from build123d import *

# Parameters (mm, degrees)
SKETCH1_W           = 150
SKETCH1_H           = 140
BOSS_EXTRUDE1_DEPTH = 10
SKETCH2_W           = 10.4
SKETCH2_H           = 41.4
CUT_EXTRUDE1_DEPTH  = 5
BOSS_EXTRUDE2_DEPTH = 150
SKETCH4_W           = 150
SKETCH4_H           = 10
SKETCH4_R           = 2
BOSS_EXTRUDE3_DEPTH = 5
SKETCH5_R           = 2
CUT_EXTRUDE2_DEPTH  = 6
SKETCH6_R           = 1.5
CUT_EXTRUDE3_DEPTH  = 5
SKETCH7_R           = 2.5
CUT_EXTRUDE4_DEPTH  = 2
SKETCH8_W           = 130
SKETCH8_H           = 120
CUT_EXTRUDE5_DEPTH  = 5
FILLET1_R           = 2.5


with BuildPart() as part:
    # Sketch1 → Boss-Extrude1 (new body)
    with BuildSketch(Plane(origin=(0, 0, 0), x_dir=(1, 0, 0), z_dir=(0, 1, 0))):
        Rectangle(SKETCH1_W, SKETCH1_H)
    extrude(amount=BOSS_EXTRUDE1_DEPTH)

    # Sketch2 → Cut-Extrude1 (cut)
    with BuildSketch(Plane.XZ):
        with Locations((-69.9, 0)):
            Rectangle(SKETCH2_W, SKETCH2_H)
        with Locations((69.9, 0)):
            Rectangle(SKETCH2_W, SKETCH2_H)
    extrude(amount=-CUT_EXTRUDE1_DEPTH, mode=Mode.SUBTRACT)

    # Sketch3 → Boss-Extrude2 (add)
    with BuildSketch(Plane.ZY.offset(75)):
        Polygon((-70, 13), (-70, 10), (-60, 10), (-60, 16), (-65, 16), align=None)
        Polygon((70, 10), (70, 13), (65, 16), (60, 16), (60, 10), align=None)
    extrude(amount=-BOSS_EXTRUDE2_DEPTH)

    # Sketch4 → Boss-Extrude3 (add)
    with BuildSketch(Plane(origin=(0, 10, 0), x_dir=(1, 0, 0), z_dir=(0, 1, 0))):
        with Locations((0, 55)):
            Rectangle(SKETCH4_W, SKETCH4_H)
        with Locations((-70, 55)):
            Circle(SKETCH4_R, mode=Mode.SUBTRACT)
        with Locations((70, 55)):
            Circle(SKETCH4_R, mode=Mode.SUBTRACT)
        with Locations((0, -55)):
            Rectangle(SKETCH4_W, SKETCH4_H)
        with Locations((70, -55)):
            Circle(SKETCH4_R, mode=Mode.SUBTRACT)
        with Locations((-70, -55)):
            Circle(SKETCH4_R, mode=Mode.SUBTRACT)
    extrude(amount=BOSS_EXTRUDE3_DEPTH)

    # Sketch5 → Cut-Extrude2 (cut)
    with BuildSketch(Plane(origin=(0, 15, 0), x_dir=(1, 0, 0), z_dir=(0, 1, 0))):
        with Locations((-70, 55)):
            Circle(SKETCH5_R)
        with Locations((70, 55)):
            Circle(SKETCH5_R)
        with Locations((-70, -55)):
            Circle(SKETCH5_R)
        with Locations((70, -55)):
            Circle(SKETCH5_R)
    extrude(amount=-CUT_EXTRUDE2_DEPTH, mode=Mode.SUBTRACT)

    # Sketch6 → Cut-Extrude3 (cut)
    with BuildSketch(Plane(origin=(0, 5, 0), x_dir=(-1, 0, 0), z_dir=(0, -1, 0))):
        with Locations((69.899999566, -11.999895835)):
            Circle(SKETCH6_R)
        with Locations((69.899999566, 11.999895835)):
            Circle(SKETCH6_R)
        with Locations((-69.899999566, -11.999895835)):
            Circle(SKETCH6_R)
        with Locations((-69.899999566, 11.999895835)):
            Circle(SKETCH6_R)
    extrude(amount=-CUT_EXTRUDE3_DEPTH, mode=Mode.SUBTRACT)

    # Sketch7 → Cut-Extrude4 (cut)
    with BuildSketch(Plane(origin=(0, 10, 0), x_dir=(1, 0, 0), z_dir=(0, 1, 0))):
        with Locations((-69.899999566, 11.999895835)):
            Circle(SKETCH7_R)
        with Locations((-69.899999566, -11.999895835)):
            Circle(SKETCH7_R)
        with Locations((69.899999566, -11.999895835)):
            Circle(SKETCH7_R)
        with Locations((69.899999566, 11.999895835)):
            Circle(SKETCH7_R)
    extrude(amount=-CUT_EXTRUDE4_DEPTH, mode=Mode.SUBTRACT)

    # Sketch8 → Cut-Extrude5 (cut)
    with BuildSketch(Plane(origin=(0, 15, 0), x_dir=(1, 0, 0), z_dir=(0, 1, 0))):
        Rectangle(SKETCH8_W, SKETCH8_H)
    extrude(amount=-CUT_EXTRUDE5_DEPTH, mode=Mode.SUBTRACT)

    # Fillet1
    fillet1_edges = [part.edges().sort_by_distance(p)[0] for p in [
        (-70, 10, 50),
        (70, 10, 50),
        (70, 10, -50),
        (65, 12.5, -50),
        (65, 10, -55),
        (65, 12.5, 50),
        (-65, 10, -55),
        (-65, 12.5, -50),
        (-65, 12.5, 50),
        (65, 10, 55),
        (-65, 10, 55),
        (-70, 10, -50),
    ]]
    fillet(fillet1_edges, radius=FILLET1_R)


solid = part.part
Geometry check sheet. Reference: the model listing, model coordinates, mm. A direction names the side the tool comes from. Round coordinates to 2 decimals unless told otherwise and drop trailing zeros. Order: outer loops, then holes, each group sorted by start corner. A loop starts at its lowest first (then second) coordinate and runs counter-clockwise, first axis right, second up. Notation, with made-up numbers: M -22,28 L -10,28 A22 cw -10,55 Z; hole C -12.75,51 d6. An arc over 180 degrees is marked long. Write each question's results on one line, items separated by ' | '. Start each with the question number.
1. Cross-section at A-A on x = -28. Record the boundary of the cut face in (y, z), plus the area to 4 significant figures.
2. Draft check along Z on faces 1 (the face through (70, 9, -55)), 2 (the face through (-1, 14.5, -67.5)), 3 (the face through (-1, 6, 70)). Enter one of: pulls with the +Z half, pulls with the -Z half, needs draft (parallel to the pull), parting line crosses it, or undercut.
3. Cross-section at B-B on z = -55. Record the boundary of the cut face in (x, y).
4. Cross-section at D-D on z = -0.5. Record the boundary of the cut face in (x, y), plus the area to 3 significant figures.
5. Set-up check for faces 4 (the face through (-67.515, 9.014, 11.249)), 5 (the face through (70, 5, 0)), 6 (the face through (69.9, 15, 57.2)), 7 (the face through (-70, 2, 20.7)): record each of +Z, -Z, +X, -X, +Y, -Y from which the full face is reachable in a straight line by a thin tool's end or side.
6. Go/stop test with flat-tipped pins: P1, Ø6, axis at y = 12, z = 48, coming from the +X side; P2, Ø3.5, axis at x = 69.9, z = 12, coming from the -Y side; P3, Ø3, axis at x = -69.5, z = 54, coming from the +Y side; P4, Ø1, axis at x = 37, z = 38.5, coming from the +Y side. Record where each tip stops, or that it passes through.
7. Material ranges on L1, parallel to Z at x = -69.9, y = 6.8; L2, parallel to X at y = 9.7, z = -55; L3, parallel to Z at x = -69.9, y = 8.75, recorded low to high. Write a range as from..to.
8. Cross-section at C-C on y = 2.5. Record the boundary of the cut face in (x, z), plus the area to 3 significant figures.
Resolved:
1) outline: M 0,-70 L 13,-70 L 16,-65 L 16,-60 L 10,-60 L 10,60 L 16,60 L 16,65 L 13,70 L 0,70 Z | area: 1,505 mm2
2) face 1: undercut | face 2: pulls with the -Z half | face 3: pulls with the +Z half
3) outline: M -75,0 L 75,0 L 75,15 L 72,15 L 72,9 L 68,9 L 68,15 L 65,15 L 65,12.5 A2.5 cw 62.5,10 L -62.5,10 A2.5 cw -65,12.5 L -65,15 L -68,15 L -68,9 L -72,9 L -72,15 L -75,15 Z
4) outline: M -75,5 L -64.7,5 L -64.7,0 L 64.7,0 L 64.7,5 L 75,5 L 75,10 L -75,10 Z | area: 1,400 mm2
5) face 4: +Y | face 5: +X, -Y | face 6: +X, -X, +Y | face 7: -X, -Y
6) P1: x = 75 | P2: y = 5 | P3: y = 15 | P4: y = 10
7) L1: -70..-13.5, -10.5..10.5, 13.5..70 | L2: -75..-72, -68..68, 72..75 | L3: -70..-14.5, -9.5..9.5, 14.5..70
8) outline: M -75,-70 L 75,-70 L 75,-20.7 L 64.7,-20.7 L 64.7,20.7 L 75,20.7 L 75,70 L -75,70 L -75,20.7 L -64.7,20.7 L -64.7,-20.7 L -75,-20.7 Z | area: 20,100 mm2
